from build123d import *

# Parameters (mm, degrees)
F0_W     = 150
F0_H     = 20
F0_R     = 2.5
F1_DEPTH = 4
F2_DEPTH = 10
F3_W     = 7.5
F3_H     = 8
F3_W_2   = 10.5527898669
F4_DEPTH = 25


# Not quite as in the source:
# - a feature names something its author has since deleted; it is built from what else it names


with BuildPart() as f1:
    # F0 (on Top) → F1 (new body, symmetric)
    with BuildSketch(Plane.XY):
        Rectangle(F0_W, F0_H)
        with BuildLine():
            Line((90, 10), (75, 10))
            Line((75, 10), (75, -10))
            Line((75, -10), (90, -10))
            ThreePointArc((90, -10), (80, 0), (90, 10))
        make_face()
        with BuildLine():
            ThreePointArc((100, 0), (97.0710678119, 7.0710678119), (90, 10))
            ThreePointArc((90, 10), (80, 0), (90, -10))
            ThreePointArc((90, -10), (97.0710678119, -7.0710678119), (100, 0))
        make_face()
        with Locations((90, 0)):
            Circle(F0_R, mode=Mode.SUBTRACT)
    extrude(amount=F1_DEPTH, both=True)

    # F0 (on Top) → F2 (join, symmetric)
    with BuildSketch(Plane.XY):
        with BuildLine():
            ThreePointArc((-80, 0), (-82.9289321881, 7.0710678119), (-90, 10))
            ThreePointArc((-90, 10), (-100, 0), (-90, -10))
            ThreePointArc((-90, -10), (-82.9289321881, -7.0710678119), (-80, 0))
        make_face()
        with Locations((-90, 0)):
            Circle(F0_R, mode=Mode.SUBTRACT)
        with BuildLine():
            Line((-75, -10), (-75, 10))
            Line((-75, 10), (-90, 10))
            ThreePointArc((-90, 10), (-82.9289321881, 7.0710678119), (-80, 0))
            ThreePointArc((-80, 0), (-82.9289321881, -7.0710678119), (-90, -10))
            Line((-90, -10), (-75, -10))
        make_face()
    extrude(amount=F2_DEPTH, both=True)

    # F3 (on face) → F4 (cut)
    with BuildSketch(Plane.XZ.offset(10)):
        with Locations((-86.25, 0)):
            Rectangle(F3_W, F3_H)
        with Locations((-95.2763949335, 0)):
            Rectangle(F3_W_2, F3_H)
    extrude(amount=-F4_DEPTH, mode=Mode.SUBTRACT)


solid = f1.part
For this review, take the finished solid that the model builds, in its own axes (mm). A direction names the side the tool comes from. Round coordinates to 2 decimals unless told otherwise and drop trailing zeros. Write each loop counter-clockwise with the first axis right and the second up, starting at its lowest first coordinate (ties: lowest second). Pieces come first, ordered by that corner, then holes. Notation, with made-up numbers: (46, -6) - (82, -6) arc R25 ccw to (82, 25) - close; hole circle Ø6 at (62.25, 40.5). An arc over 180 degrees is marked (long way). Write item = value, one per line. Start each with the question number.
1. For faces 1 (the face through (-75, 0, -7)), 2 (the face through (11, 0, 4)), 3 (the face through (-93, 0, 4)), list the 3-axis set-ups (+Z, -Z, +X, -X, +Y, -Y) from which the entire face can be reached by the end or side of a thin tool; tool diameter is ignored.
2. Consider section C-C on x = 63. State the section outline as (y, z) points.
3. Consider section A-A on y = 0. State the section outline as (x, z) points.
4. Draft analysis for pull direction X (two halves, no side actions). For faces 4 (the face through (87.5, 0.1, -0.1)), 5 (the face through (-21, -10, 0)), 6 (the face through (-82.5, 0, 0)), state which applies: released by +X, released by -X, zero draft, split by the parting line, or undercut.
5. For pin 1 Ø8 at (y, z) = (7, -3.5) entering from +X; pin 2 Ø6.5 at (y, z) = (5, 6) entering from +X; pin 3 Ø3 at (x, y) = (-45, 6.5) entering from -Z; pin 4 Ø12 at (x, z) = (-8, -6.5) entering from -Y, all flat-tipped, find the tip position at first contact; note any pin that passes through.
6. Wall thickness on L1, parallel to X at y = 0, z = 5.3; L2, parallel to Y at x = -90, z = -8.3; L3, parallel to Z at x = -84.5, y = 9: over which ranges is each line inside the solid? List them lowest first.
7. Consider section B-B on z = -8. State the section outline as (x, y) points, plus the area to 3 significant figures.
Evaluation:
q1.face_1 = -Z, +X, +Y, -Y
q1.face_2 = +Z, +X, +Y, -Y
q1.face_3 = -X, +Y, -Y
q2.outline = (-10, -4) - (10, -4) - (10, 4) - (-10, 4) - close
q3.outline = (-100, -10) - (-92.5, -10) - (-92.5, -4) - (-100, -4) - close; (-100, 4) - (-92.5, 4) - (-92.5, 10) - (-100, 10) - close; (-87.5, -10) - (-75, -10) - (-75, -4) - (87.5, -4) - (87.5, 4) - (-75, 4) - (-75, 10) - (-87.5, 10) - (-87.5, 4) - (-82.5, 4) - (-82.5, -4) - (-87.5, -4) - close; (92.5, -4) - (100, -4) - (100, 4) - (92.5, 4) - close
q4.face_4 = undercut
q4.face_5 = zero draft
q4.face_6 = released by -X
q5.pin_1 = 99.54
q5.pin_2 = 99.7
q5.pin_3 = -4
q5.pin_4 = -10
q6.L1 = -100 to -92.5, -87.5 to -75
q6.L2 = -10 to -2.5, 2.5 to 10
q6.L3 = -10 to -4, 4 to 10
q7.outline = (-90, -10) - (-75, -10) - (-75, 10) - (-90, 10) arc R10 ccw to start; hole circle Ø5 at (-90, 0)
q7.area = 437 mm2
